Input: part model. Units: mm. Frame: model coordinates. A direction names the side the tool comes from. Round coordinates to 2 decimals unless told otherwise and drop trailing zeros. Write each loop counter-clockwise with the first axis right and the second up, starting at its lowest first coordinate (ties: lowest second). Pieces come first, ordered by that corner, then holes. Notation, with made-up numbers: (87.5, -8.5) - (115.5, -8.5) arc R19 cw to (115.5, 10.5) - close; hole circle Ø3 at (-18, -8). An arc over 180 degrees is marked (long way). One line per item, written item: value. Start each with the question number.
```python
from build123d import *

# Parameters (mm, degrees)
F1_DEPTH = 3
F2_R     = 4.5
F2_R_2   = 2.5
F3_DEPTH = 5


with BuildPart() as f1:
    # F0 (on Top) → F1 (new body)
    with BuildSketch(Plane.XY):
        with BuildLine():
            Line((-15, -20), (15, -20))
            ThreePointArc((15, -20), (29.142136, -14.142136), (35, 0))
            ThreePointArc((35, 0), (29.142136, 14.142136), (15, 20))
            Line((15, 20), (-15, 20))
            ThreePointArc((-15, 20), (-29.142136, 14.142136), (-35, 0))
            ThreePointArc((-35, 0), (-29.142136, -14.142136), (-15, -20))
        make_face()
    extrude(amount=F1_DEPTH)

    # F2 (on face) → F3 (join)
    with BuildSketch(Plane.XY.offset(3)):
        with Locations((-15, 0)):
            Circle(F2_R)
        with Locations((-15, 0)):
            Circle(F2_R_2, mode=Mode.SUBTRACT)
        with Locations((15, 0)):
            Circle(F2_R)
        with Locations((15, 0)):
            Circle(F2_R_2, mode=Mode.SUBTRACT)
    extrude(amount=F3_DEPTH)


solid = f1.part
```
Q1. Cut plane C-C, the plane x = -1. Output: boundary loops of the cut face in (y, z), and give its area (3 significant figures).
Q2. Access query for faces 1 (the flat face through (0, -20, 1)), 2 (the cylindrical face through (12.5, 0.1, 5.5)). Directions: +Z, -Z, +X, -X, +Y, -Y. A direction counts if a zero-diameter tool reaches every point of the face in a straight line with its end or side. Return the directions, or none.
Q3. Cut plane A-A, the plane y = -3.5. Output: boundary loops of the cut face in (x, z).
Q4. Contact query for flat-ended pins moving along their axis: pin 1 Ø1.5 at (x, y) = (-16, -0.5) entering from +Z; pin 2 Ø1.5 at (x, z) = (20.5, 3.5) entering from -Y. Output: stop coordinate, or through.
Q5. Pull-direction query (Y, two-part tool) for faces 3 (the flat face through (0, 20, 1)), 4 (the flat face through (0, 0, 3)), 5 (the flat face through (-15, 0, 3)); classes: pulls with the +Y half, pulls with the -Y half, needs draft (parallel to the pull), parting line crosses it, or undercut.
Q6. Cut plane D-D, the plane y = 11. Output: boundary loops of the cut face in (x, z), and give its area (3 significant figures).
Q7. Material intervals for probe 1 along X at (y, z) = (-1.5, 5); probe 2 along Z at (x, y) = (-31.5, 9); probe 3 along X at (y, z) = (-1, 5.5), sorted ascending. Write a range as from..to.
Q8. Cut plane B-B, the plane x = 11.5. Output: boundary loops of the cut face in (y, z), and give its area (3 significant figures).
A:
1. outline: (-20, 0) - (20, 0) - (20, 3) - (-20, 3) - close
1. area: 120 mm²
2. face 1: +Z, -Z, +X, -X, -Y
2. face 2: +Z
3. outline: (-34.69, 0) - (34.69, 0) - (34.69, 3) - (17.83, 3) - (17.83, 8) - (12.17, 8) - (12.17, 3) - (-12.17, 3) - (-12.17, 8) - (-17.83, 8) - (-17.83, 3) - (-34.69, 3) - close
4. pin 1: stops at z = 3
4. pin 2: stops at y = -19.38
5. face 3: pulls with the +Y half
5. face 4: needs draft
5. face 5: undercut
6. outline: (-31.7, 0) - (31.7, 0) - (31.7, 3) - (-31.7, 3) - close
6. area: 190 mm²
7. probe 1: x = -19.24..-17, -13..-10.76, 10.76..13, 17..19.24
7. probe 2: z = 0..3
7. probe 3: x = -19.39..-17.29, -12.71..-10.61, 10.61..12.71, 17.29..19.39
8. outline: (-20, 0) - (20, 0) - (20, 3) - (2.83, 3) - (2.83, 8) - (-2.83, 8) - (-2.83, 3) - (-20, 3) - close
8. area: 148 mm²
